Geometry check sheet. Reference: the model listing, model coordinates, mm. A direction names the side the tool comes from. Coordinates: 2 decimals unless noted, no trailing zeros. Order: outer loops, then holes, each group sorted by start corner. A loop starts at its lowest first (then second) coordinate and runs counter-clockwise, first axis right, second up. Notation, with made-up numbers: (27, 45.25) - (44, 45.25) arc R16 ccw to (44, 56.25) - close; hole circle Ø4 at (11.5, 63.25). An arc over 180 degrees is marked (long way). Put each result on its own line as item: value.
from build123d import *

# Parameters (mm, degrees)
SKETCH1_W           = 27.9
SKETCH1_H           = 20.08
SKETCH1_W_2         = 25.9
SKETCH1_H_2         = 18.08
BOSS_EXTRUDE1_DEPTH = 10
SKETCH3_W           = 27.5
SKETCH3_H           = 19.88
BOSS_EXTRUDE2_DEPTH = 1
SKETCH4_R           = 1.15
BOSS_EXTRUDE3_DEPTH = 10
SKETCH12_R          = 3
BOSS_EXTRUDE6_DEPTH = 6


with BuildPart() as part:
    # Sketch1 → Boss-Extrude1 (new body)
    with BuildSketch(Plane(origin=(0, 0, 0), x_dir=(1, 0, 0), z_dir=(0, 1, 0))):
        Rectangle(SKETCH1_W, SKETCH1_H)
        Rectangle(SKETCH1_W_2, SKETCH1_H_2, mode=Mode.SUBTRACT)
    extrude(amount=BOSS_EXTRUDE1_DEPTH)

    # Sketch3 → Boss-Extrude2 (add)
    with BuildSketch(Plane(origin=(0, 0, 0), x_dir=(1, 0, 0), z_dir=(0, 1, 0))):
        Rectangle(SKETCH3_W, SKETCH3_H)
    extrude(amount=-BOSS_EXTRUDE2_DEPTH)

    # Sketch4 → Boss-Extrude3 (add)
    with BuildSketch(Plane(origin=(0, 0, 0), x_dir=(1, 0, 0), z_dir=(0, 1, 0))):
        with Locations(Location((-10.16, 6.35, 0), (0, 0, 270))):
            Circle(SKETCH4_R)
        with Locations(Location((10.16, 6.35, 0), (0, 0, 270))):
            Circle(SKETCH4_R)
        with Locations(Location((-10.16, -6.35, 0), (0, 0, 270))):
            Circle(SKETCH4_R)
        with Locations(Location((10.16, -6.35, 0), (0, 0, 270))):
            Circle(SKETCH4_R)
    extrude(amount=BOSS_EXTRUDE3_DEPTH)

    # Sketch12 → Boss-Extrude6 (add)
    # profile 1 of 4: a face of its own
    with BuildSketch(Plane(origin=(40.87798925, -1, 20.164210109), x_dir=(-1, 0, 0), z_dir=(0, -1, 0))):
        with BuildLine():
            Line((27.12798925, 35.104210109), (27.12798925, 30.104210109))
            Line((27.12798925, 30.104210109), (37.12798925, 30.104210109))
            Line((37.12798925, 30.104210109), (37.12798925, 35.104210109))
            ThreePointArc((37.12798925, 35.104210109), (32.12798925, 40.104210109), (27.12798925, 35.104210109))
        make_face()
        with Locations(Location((32.12798925, 35.104210109, 0), (0, 0, 90))):
            Circle(SKETCH12_R, mode=Mode.SUBTRACT)
    # profile 2 of 4: a face of its own
    with BuildSketch(Plane(origin=(40.87798925, -1, 20.164210109), x_dir=(-1, 0, 0), z_dir=(0, -1, 0))):
        with BuildLine():
            Line((37.12798925, 5.224210109), (37.12798925, 10.224210109))
            Line((37.12798925, 10.224210109), (27.12798925, 10.224210109))
            Line((27.12798925, 10.224210109), (27.12798925, 5.224210109))
            ThreePointArc((27.12798925, 5.224210109), (32.12798925, 0.224210109), (37.12798925, 5.224210109))
        make_face()
        with Locations(Location((32.12798925, 5.224210109, 0), (0, 0, 90))):
            Circle(SKETCH12_R, mode=Mode.SUBTRACT)
    # profile 3 of 4: a face of its own
    with BuildSketch(Plane(origin=(40.87798925, -1, 20.164210109), x_dir=(-1, 0, 0), z_dir=(0, -1, 0))):
        with BuildLine():
            Line((54.62798925, 5.224210109), (54.62798925, 10.224210109))
            Line((54.62798925, 10.224210109), (44.62798925, 10.224210109))
            Line((44.62798925, 10.224210109), (44.62798925, 5.224210109))
            ThreePointArc((44.62798925, 5.224210109), (49.62798925, 0.224210109), (54.62798925, 5.224210109))
        make_face()
        with Locations(Location((49.62798925, 5.224210109, 0), (0, 0, 90))):
            Circle(SKETCH12_R, mode=Mode.SUBTRACT)
    # profile 4 of 4: a face of its own
    with BuildSketch(Plane(origin=(40.87798925, -1, 20.164210109), x_dir=(-1, 0, 0), z_dir=(0, -1, 0))):
        with BuildLine():
            Line((44.62798925, 35.104210109), (44.62798925, 30.104210109))
            Line((44.62798925, 30.104210109), (54.62798925, 30.104210109))
            Line((54.62798925, 30.104210109), (54.62798925, 35.104210109))
            ThreePointArc((54.62798925, 35.104210109), (49.62798925, 40.104210109), (44.62798925, 35.104210109))
        make_face()
        with Locations(Location((49.62798925, 35.104210109, 0), (0, 0, 90))):
            Circle(SKETCH12_R, mode=Mode.SUBTRACT)
    extrude(amount=-BOSS_EXTRUDE6_DEPTH)


solid = part.part
Q1. Section check B-B on y = 6.75. Record the boundary of the cut face in (x, z).
Answer block:
outline: (-13.95, -10.04) - (13.95, -10.04) - (13.95, 10.04) - (-13.95, 10.04) - close; circle Ø2.3 at (-10.16, -6.35); circle Ø2.3 at (-10.16, 6.35); circle Ø2.3 at (10.16, -6.35); circle Ø2.3 at (10.16, 6.35); hole (-12.95, -9.04) - (12.95, -9.04) - (12.95, 9.04) - (-12.95, 9.04) - close
Q2. Thickness scan on L1, parallel to X at y = 2.35, z = 14.94; L2, parallel to Z at x = 6.5, y = 7. Record the ranges inside material, lowest first. Write a range as [from, to].
Answer block:
L1: x = [-13.75, -11.75], [-5.75, -3.75], [3.75, 5.75], [11.75, 13.75]
L2: z = [-10.04, -9.04], [9.04, 10.04]
Q3. Section check C-C on x = 2.5. Record the boundary of the cut face in (y, z), then the cut area to 3 significant figures.
Answer block:
outline: (-1, -9.94) - (0, -9.94) - (0, -10.04) - (10, -10.04) - (10, -9.04) - (0, -9.04) - (0, 9.04) - (10, 9.04) - (10, 10.04) - (0, 10.04) - (0, 9.94) - (-1, 9.94) - close
area: 39.9 mm^2
Q4. Section check A-A on y = 1.25. State how many separate pieces and enclosed holes the cut face has, then the cut area to 3 significant figures.
Answer block:
separate pieces: 5
enclosed holes: 5
area: 349 mm^2
Q5. Section check D-D on z = -16.5. Record the boundary of the cut face in (x, y).
Answer block:
outline: (-13.5, -1) - (-11.31, -1) - (-11.31, 5) - (-13.5, 5) - close; (-6.19, -1) - (-4, -1) - (-4, 5) - (-6.19, 5) - close; (4, -1) - (6.19, -1) - (6.19, 5) - (4, 5) - close; (11.31, -1) - (13.5, -1) - (13.5, 5) - (11.31, 5) - close
Q6. Access from +Z, -Z, +X, -X, +Y, -Y to the whole of each face (thin tool, end or side, straight path). Record for faces 3 (the flat face through (-8.7, 5, 11.6)), 4 (the cylindrical face through (-8.64, 1.96, 19.94)), 5 (the flat face through (0, 0, 0)).
Answer block:
face 3: +Z, +X, -X, +Y
face 4: +Z, +Y, -Y
face 5: +Y
Q7. Depth check by flat-ended pin: pin 1 Ø8 at (x, z) = (10, -17) entering from +Y; pin 2 Ø2.5 at (y, z) = (1, -13.5) entering from -X; pin 3 Ø4 at (x, z) = (-6.5, 4.5) entering from +Y. Enter the tip coordinate at first touch or a pass-through.
Answer block:
pin 1: stops at y = 5
pin 2: stops at x = -13.75
pin 3: stops at y = 0
Q8. Draft check along X on faces 1 (the cylindrical face through (-11.283, 4.93, -6.599)), 2 (the flat face through (8.8, 5, 11.6)). Enter one of: pulls with the +X half, pulls with the -X half, needs draft (parallel to the pull), parting line crosses it, or undercut.
Answer block:
face 1: undercut
face 2: needs draft
